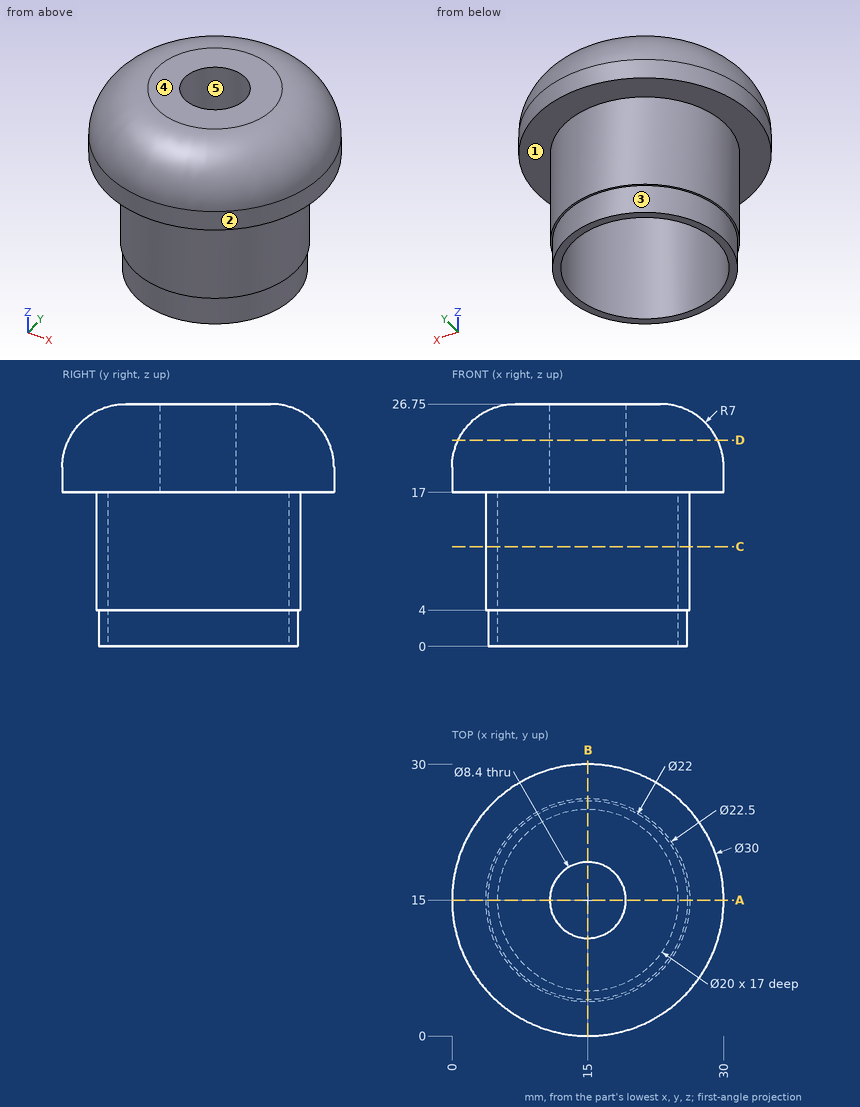
Input: dimensioned drawing with shaded views. Units: mm. Origin: part minimum x, y, z. A direction names the side the tool comes from. Coordinates: 2 decimals unless noted, no trailing zeros. Loops run counter-clockwise (first coordinate to the right, second up) from the corner with the lowest first, then second, coordinate; pieces in that order, holes last. Notation, with made-up numbers: M 18.25,50 L 42.25,50 A28 ccw 42.25,72 Z; hole C 83.5,-25.5 d1. An arc over 180 degrees is marked long. Use a Markdown table: item, result. Add a question column.
Q1. Access query for the marked faces 1 and 2. Directions: +Z, -Z, +X, -X, +Y, -Y. A direction counts if a zero-diameter tool reaches every point of the face in a straight line with its end or side. Return the directions, or none.
Q2. Draft query along Y for the marked faces 3, 4 and 5. Return one class per face: pulls with the +Y half, pulls with the -Y half, needs draft (parallel to the pull), parting line crosses it, or undercut.
Q3. Section query C-C, the plane z = 11. Return loops of the section in (x, y), and give its area (3 significant figures).
Q4. Section query A-A, the plane y = 15. Return loops of the section in (x, z).
Q5. Section query D-D, the plane z = 22.75. Return loops of the section in (x, y), and give its area (3 significant figures).
Q6. First-contact query: pin 1 (2 mm diameter, centred on x = 5.5, z = 21, fed in from -Y); pin 2 (10 mm diameter, centred on x = 6, z = 3, fed in from +Y); pin 3 (2 mm diameter, centred on x = 18.5, z = 5.5, fed in from -Y). Flat tips, straight axial feed; report the tip coordinate or a pass-through.
Q7. Material intervals for L1, parallel to Y at x = 15, z = 12.5; L2, parallel to Y at x = 15, z = 19.5; L3, parallel to X at y = 19.5, z = 5, sorted ascending.
Result:
| question | item | result |
|---|---|---|
| 1 | face 1 | -Z |
| 1 | face 2 | +Z, -Z |
| 2 | face 3 | parting line crosses it |
| 2 | face 4 | needs draft |
| 2 | face 5 | undercut |
| 3 | outline | C 15,15 d22.5; hole C 15,15 d20 |
| 3 | area | 83.4 mm2 |
| 4 | outline | M 0,17 L 3.75,17 L 3.75,4 L 4,4 L 4,0 L 5,0 L 5,17 L 10.8,17 L 10.8,26.75 L 7,26.75 A7 ccw 0,19.75 Z; M 19.2,17 L 25,17 L 25,0 L 26,0 L 26,4 L 26.25,4 L 26.25,17 L 30,17 L 30,19.75 A7 ccw 23,26.75 L 19.2,26.75 Z |
| 5 | outline | C 15,15 d28.65; hole C 15,15 d8.4 |
| 5 | area | 589 mm2 |
| 6 | pin 1 | stops at y = 2.75 |
| 6 | pin 2 | stops at y = 25.48 |
| 6 | pin 3 | stops at y = 4.03 |
| 7 | L1 | y = 3.75 to 5, 25 to 26.25 |
| 7 | L2 | y = 0 to 10.8, 19.2 to 30 |
| 7 | L3 | x = 4.69 to 6.07, 23.93 to 25.31 |
